The figure shows three views and two pictorial views of one solid part (mm, origin at its lowest corner). Answer the questions. Round coordinates to 2 decimals unless told otherwise and drop trailing zeros. Write each loop counter-clockwise with the first axis right and the second up, starting at its lowest first coordinate (ties: lowest second). Pieces come first, ordered by that corner, then holes.
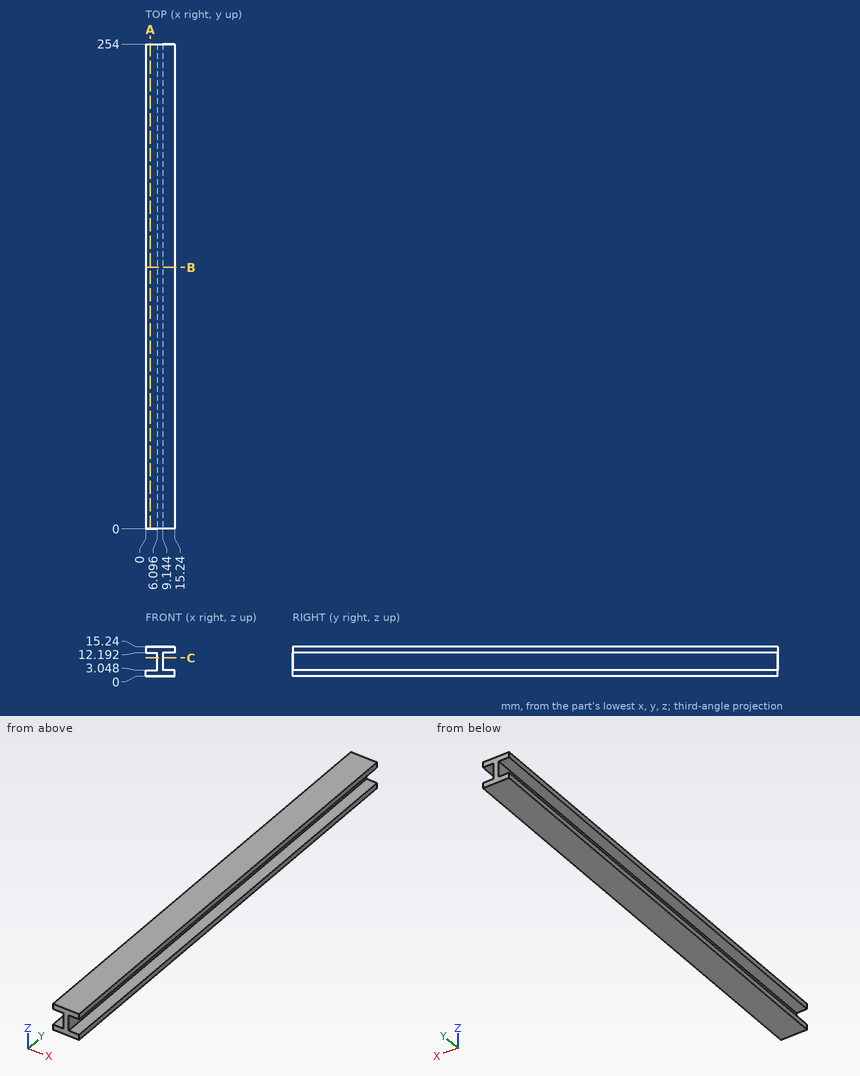
Q1. Straight lines are drawn through the part: probe 1 along Z at (x, y) = (10, 212.5); probe 2 along X at (y, z) = (150, 8.5). For each, find the intervals that lie inside material, in ascending order.
Verdict:
probe 1: z = 0 to 3.05, 12.19 to 15.24
probe 2: x = 6.1 to 9.14
Q2. Section B-B (y = 137) is taken. Determine the outline of the cut face in (x, z), then the cut area to 3 significant figures.
Verdict:
outline: (0, 0) - (15.24, 0) - (15.24, 3.05) - (9.14, 3.05) - (9.14, 12.19) - (15.24, 12.19) - (15.24, 15.24) - (0, 15.24) - (0, 12.19) - (6.1, 12.19) - (6.1, 3.05) - (0, 3.05) - close
area: 121 mm2
Q3. Flat-ended cylindrical pins translate along their axes: pin 1 Ø8 at (x, z) = (11.5, 5.5) entering from +Y; pin 2 Ø3 at (y, z) = (68, 9) entering from +X; pin 3 Ø2 at (y, z) = (148, 8.5) entering from -X; pin 4 Ø1 at (x, z) = (3.5, 5.5) entering from +Y. Find the tip coordinate at first contact, or state that the pin passes through.
Verdict:
pin 1: stops at y = 254
pin 2: stops at x = 9.14
pin 3: stops at x = 6.1
pin 4: passes through
Q4. Section C-C (z = 9.5) is taken. Determine the outline of the cut face in (x, y), then the cut area to 3 significant figures.
Verdict:
outline: (6.1, 0) - (9.14, 0) - (9.14, 254) - (6.1, 254) - close
area: 774 mm2
Q5. Section A-A (x = 2.5) is taken. Determine the outline of the cut face in (y, z), then the cut area to 3 significant figures.
Verdict:
outline: (0, 0) - (254, 0) - (254, 3.05) - (0, 3.05) - close; (0, 12.19) - (254, 12.19) - (254, 15.24) - (0, 15.24) - close
area: 1,550 mm2
